Design review of the part built by this model. Coordinates are the model's own, in mm. Coordinates: 2 decimals unless noted, no trailing zeros. Write each loop counter-clockwise with the first axis right and the second up, starting at its lowest first coordinate (ties: lowest second). Pieces come first, ordered by that corner, then holes. Notation, with made-up numbers: (84, -5.75) - (93, -5.75) arc R15 cw to (93, 2.25) - close; hole circle Ø4 at (-34, -29.5). An arc over 180 degrees is marked (long way). One line per item, written item: value.
from build123d import *

# Parameters (mm, degrees)
AUFSATZ_LINEAR_AUSTRAGEN1_DEPTH = 3.5


with BuildPart() as part:
    # Skizze1 → Aufsatz-Linear austragen1 (new body, symmetric)
    with BuildSketch(Plane.XY):
        with BuildLine():
            Line((831.647452371, 366.448530177), (628.572821229, 366.448530177))
            Line((628.572821229, 366.448530177), (628.572821229, 375.106989994))
            Line((628.572821229, 375.106989994), (274.428895499, 375.106989994))
            add(Edge.make_bspline(
                [(274.428895499, 375.106989994), (256.358547924, 375.106989994), (247.122592497, 394.383569374)],
                knots=[0, 0, 0, 1, 1, 1], degree=2))
            Line((247.122592497, 394.383569374), (174.038075638, 369.085082769))
            add(Edge.make_bspline(
                [(174.038075638, 369.085082769), (207.417770849, 336.709288166), (244.126187853, 323.555937748), (280.251563051, 322.503742353)],
                knots=[0, 0, 0, 0, 1, 1, 1, 1], degree=3))
            Line((280.251563051, 322.503742353), (527.843524378, 322.503742353))
            add(Edge.make_bspline(
                [(527.843524378, 322.503742353), (541.993033664, 322.503742353), (557.358077917, 311.262922103), (560.616559045, 310.285377764)],
                knots=[0, 0, 0, 0, 1, 1, 1, 1], degree=3))
            add(Edge.make_bspline(
                [(560.616559045, 310.285377764), (569.016239065, 321.364266067), (579.47275725, 327.823555694), (591.986113601, 329.663246645)],
                knots=[0, 0, 0, 0, 1, 1, 1, 1], degree=3))
            add(Edge.make_bspline(
                [(591.986113601, 329.663246645), (599.533888677, 330.772906845), (610.017065826, 327.93253872), (610.038691557, 327.93253872)],
                knots=[0, 0, 0, 0, 1, 1, 1, 1], degree=3))
            Line((610.038691557, 327.93253872), (628.174793789, 327.93253872))
            Line((628.174793789, 327.93253872), (628.174793789, 336.911119919))
            Line((628.174793789, 336.911119919), (846.52672127, 336.911119919))
            Line((846.52672127, 336.911119919), (831.647452371, 366.448530177))
        make_face()
    extrude(amount=AUFSATZ_LINEAR_AUSTRAGEN1_DEPTH, both=True)


solid = part.part
1. Wall thickness on line 1 along Y through (x, z) = (648.5, 0.75); line 2 along Y through (x, z) = (621, -0.5); line 3 along X through (y, z) = (363.5, 0.5): over which ranges is each line inside the solid? List them lowest first.
Answer block:
line 1: y = 336.91 to 366.45
line 2: y = 327.93 to 375.11
line 3: x = 180.04 to 833.13
2. Consider section B-B, the plane x = 388. Write out the cut boundary in (y, z), then the cut area to 3 significant figures.
Answer block:
outline: (322.5, -3.5) - (375.11, -3.5) - (375.11, 3.5) - (322.5, 3.5) - close
area: 368 mm^2
3. Consider section A-A, the plane x = 715. Write out the cut boundary in (y, z), then the cut area to 3 significant figures.
Answer block:
outline: (336.91, -3.5) - (366.45, -3.5) - (366.45, 3.5) - (336.91, 3.5) - close
area: 207 mm^2
4. Insertion check: pin 1 Ø2 at (x, z) = (713, 0) entering from +Y; pin 2 Ø3 at (x, z) = (607.5, 1) entering from +Y; pin 3 Ø3 at (y, z) = (350.5, 1.5) entering from -X. Each pin has a flat end and moves straight along its axis. Give the tip position at first contact, or say it passes through.
Answer block:
pin 1: stops at y = 366.45
pin 2: stops at y = 375.11
pin 3: stops at x = 194.31
